For this review, use the dimensioned drawing (mm, ordinates from the lowest corner) and the shaded views. A direction names the side the tool comes from. Coordinates: 2 decimals unless noted, no trailing zeros. Write each loop counter-clockwise with the first axis right and the second up, starting at its lowest first coordinate (ties: lowest second). Pieces come first, ordered by that corner, then holes.
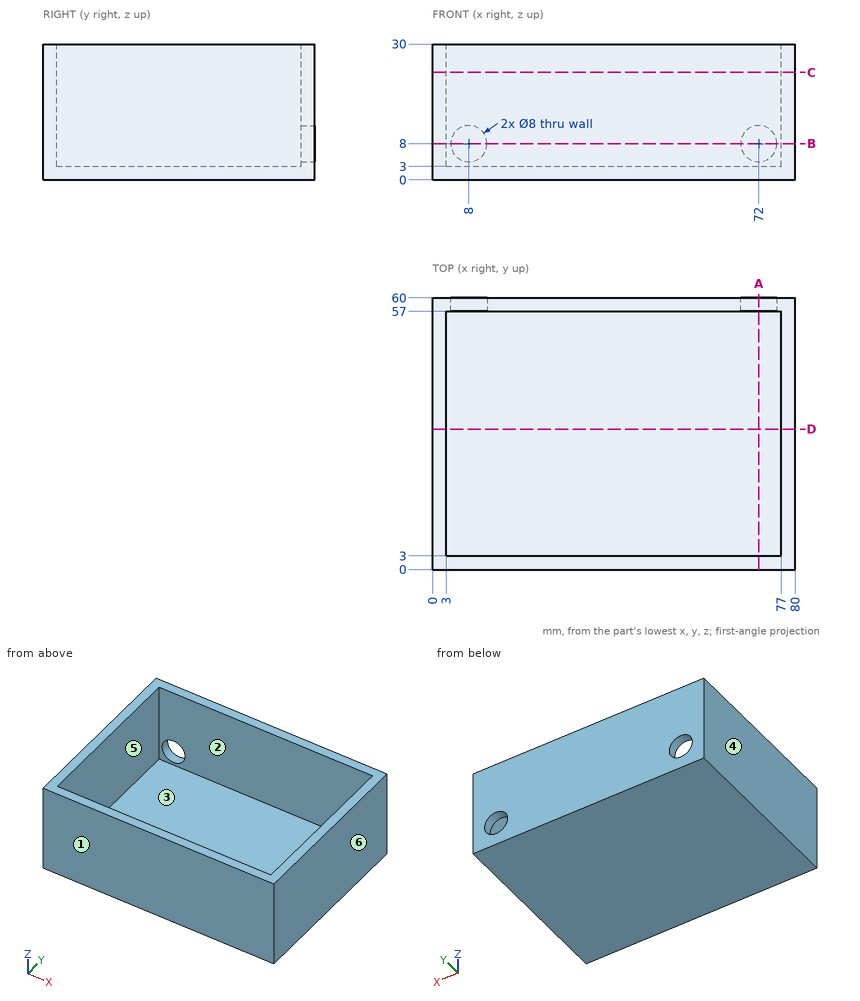
Item 1: Take a section at D-D, the plane y = 31. Write out the cut boundary in (x, z).
Solved:
outline: (0, 0) - (80, 0) - (80, 30) - (77, 30) - (77, 3) - (3, 3) - (3, 30) - (0, 30) - close
Item 2: For pin 1 (3 mm diameter, centred on x = 17.5, y = 12.5, fed in from -Z); pin 2 (5 mm diameter, centred on x = 8, z = 8, fed in from +Y), all flat-tipped, find the tip position at first contact; note any pin that passes through.
Solved:
pin 1: stops at z = 0
pin 2: stops at y = 3
Item 3: Take a section at B-B, the plane z = 8. Write out the cut boundary in (x, y), plus the area to 3 significant figures.
Solved:
outline: (0, 0) - (80, 0) - (80, 60) - (76, 60) - (76, 57) - (77, 57) - (77, 3) - (3, 3) - (3, 57) - (4, 57) - (4, 60) - (0, 60) - close; (12, 57) - (68, 57) - (68, 60) - (12, 60) - close
area: 756 mm2
Item 4: Take a section at A-A, the plane x = 72. Write out the cut boundary in (y, z), plus the area to 3 significant figures.
Solved:
outline: (0, 0) - (60, 0) - (60, 4) - (57, 4) - (57, 3) - (3, 3) - (3, 30) - (0, 30) - close; (57, 12) - (60, 12) - (60, 30) - (57, 30) - close
area: 318 mm2
Item 5: Machinability: for the marked faces 5 and 6, which of the approach directions +Z, -Z, +X, -X, +Y, -Y give a long, thin tool a straight path to every point of the face, cutting with its end or side? Answer none if there is none.
Solved:
face 5: +Z
face 6: +Z, -Z, +X, +Y, -Y
Item 6: Mouldability with a two-part tool opening along Y and no side actions: class the marked faces 1, 2, 3 and 4 as pulls with the +Y half, pulls with the -Y half, needs draft (parallel to the pull), parting line crosses it, or undercut.
Solved:
face 1: pulls with the -Y half
face 2: undercut
face 3: undercut
face 4: needs draft
Item 7: To check wall thickness, follow line 1 along X through (y, z) = (59.05, 8); line 2 along X through (y, z) = (39, 13.5); line 3 along Z through (x, y) = (8, 58). State the ranges of each line that lie inside material, in increasing order.
Solved:
line 1: x = 0 to 4, 12 to 68, 76 to 80
line 2: x = 0 to 3, 77 to 80
line 3: z = 0 to 4, 12 to 30
Item 8: Take a section at C-C, the plane z = 23.75. Write out the cut boundary in (x, y).
Solved:
outline: (0, 0) - (80, 0) - (80, 60) - (0, 60) - close; hole (3, 3) - (77, 3) - (77, 57) - (3, 57) - close
